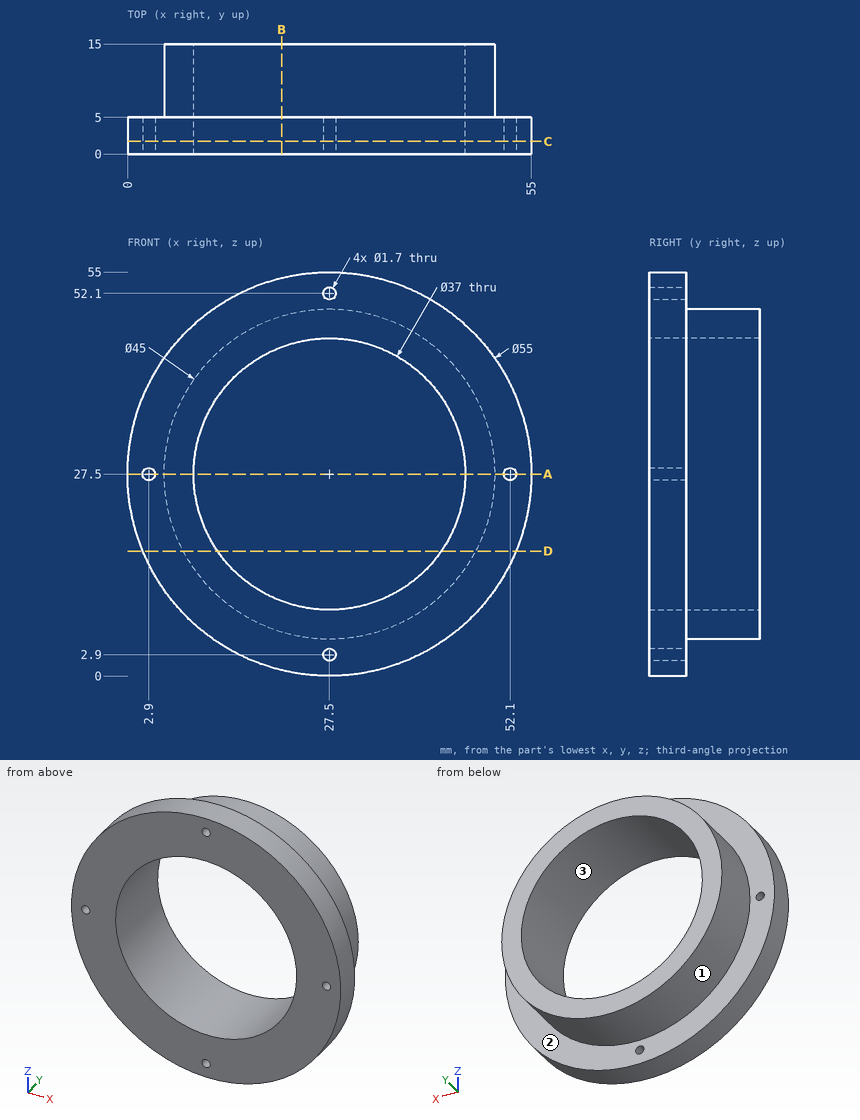
Job drawing, mm, ordinate dimensions from the low corner. One solid piece. Give positions to 0.01 mm unless a question says otherwise; leave off trailing zeros. Loops run counter-clockwise (first coordinate to the right, second up) from the corner with the lowest first, then second, coordinate; pieces in that order, holes last. Notation, with made-up numbers: M 18,18.25 L 45,18.25 A30 cw 45,56.25 Z; hole C 52,80 d3. An arc over 180 degrees is marked long. Use one line per item in the form item = value.
Item 1: Slice it at D-D on z = 17. List the corners of the cut face in (x, y).
Filled in:
outline = M 2.08,0 L 12.27,0 L 12.27,15 L 7.6,15 L 7.6,5 L 2.08,5 Z; M 42.73,0 L 52.92,0 L 52.92,5 L 47.4,5 L 47.4,15 L 42.73,15 Z
Item 2: Flat gauge pins, fed straight in: pin 1 Ø3 at (x, y) = (23, 2) entering from -Z; pin 2 Ø4 at (y, z) = (9, 26) entering from -X; pin 3 Ø3 at (y, z) = (11, 36.5) entering from +X. Where does each tip first touch, or does it go through?
Filled in:
pin_1 = 0.16
pin_2 = 5
pin_3 = 48.71
Item 3: Slice it at C-C on y = 1.75. List the corners of the cut face in (x, z), and give its area (3 significant figures).
Filled in:
outline = C 27.5,27.5 d55; hole C 2.9,27.5 d1.7; hole C 27.5,27.5 d37; hole C 27.5,2.9 d1.7; hole C 27.5,52.1 d1.7; hole C 52.1,27.5 d1.7
area = 1,290 mm^2
Item 4: Drill centre lines: L1, parallel to X at y = 2.1, z = 27.5; L2, parallel to X at y = 2.3, z = 52.1; L3, parallel to X at y = 5.25, z = 30. Where is each one in solid material? Low to high.
Filled in:
L1 = 0 to 2.05, 3.75 to 9, 46 to 51.25, 52.95 to 55
L2 = 15.21 to 26.65, 28.35 to 39.79
L3 = 5.14 to 9.17, 45.83 to 49.86
Item 5: Slice it at A-A on z = 27.5. List the corners of the cut face in (x, y).
Filled in:
outline = M 0,0 L 2.05,0 L 2.05,5 L 0,5 Z; M 3.75,0 L 9,0 L 9,15 L 5,15 L 5,5 L 3.75,5 Z; M 46,0 L 51.25,0 L 51.25,5 L 50,5 L 50,15 L 46,15 Z; M 52.95,0 L 55,0 L 55,5 L 52.95,5 Z
Item 6: Two-plate mould, pull along Z, no slides. Class the marked faces 1, 2 and 3: released by +Z, released by -Z, zero draft, split by the parting line, or undercut.
Filled in:
face_1 = split by the parting line
face_2 = zero draft
face_3 = undercut
Item 7: Slice it at B-B on x = 21. List the corners of the cut face in (y, z), and give its area (3 significant figures).
Filled in:
outline = M 0,0.78 L 5,0.78 L 5,5.96 L 15,5.96 L 15,10.18 L 0,10.18 Z; M 0,44.82 L 15,44.82 L 15,49.04 L 5,49.04 L 5,54.22 L 0,54.22 Z
area = 178 mm^2
